Geometry check sheet. Reference: the model listing, model coordinates, mm. Coordinates: 2 decimals unless noted, no trailing zeros. Write each loop counter-clockwise with the first axis right and the second up, starting at its lowest first coordinate (ties: lowest second). Pieces come first, ordered by that corner, then holes.
from build123d import *

# Parameters (mm, degrees)
BOSS_EXTRUDE1_DEPTH     = 15
CUT_EXTRUDE1_DEPTH      = 30.681644159
CUT_EXTRUDE1_DEPTH_BACK = 30.681644159
SKETCH3_R               = 2.05


with BuildPart() as part:
    # Sketch2 → Boss-Extrude1 (new body)
    with BuildSketch(Plane(origin=(0, 0, 0), x_dir=(1, 0, 0), z_dir=(0, 1, 0))):
        with BuildLine():
            Line((-16, 20), (16, 20))
            Line((16, 20), (16, 0))
            Line((16, 0), (9.075, 0))
            ThreePointArc((9.075, 0), (0, 9.075), (-9.075, 0))
            Line((-9.075, 0), (-16, 0))
            Line((-16, 0), (-16, 20))
        make_face()
    extrude(amount=BOSS_EXTRUDE1_DEPTH)

    # Sketch3 → Cut-Extrude1 (cut, two sides: drawn at the far end of the back side and taken through both)
    with BuildSketch(Plane(origin=(0, 0, -20), x_dir=(-1, 0, 0), z_dir=(0, 0, -1)).offset(-CUT_EXTRUDE1_DEPTH_BACK)):
        with Locations((-12.75, 7.5)):
            Circle(SKETCH3_R)
        with Locations((12.75, 7.5)):
            Circle(SKETCH3_R)
    extrude(amount=CUT_EXTRUDE1_DEPTH + CUT_EXTRUDE1_DEPTH_BACK, mode=Mode.SUBTRACT)


solid = part.part
1. Draft check along X on faces 1 (the flat face through (-16, 7, -10)), 2 (the flat face through (0, 0, -12)), 3 (the cylindrical face through (0.2, 7.395, -9.073)). Enter one of: released by +X, released by -X, zero draft, split by the parting line, or undercut.
Computed values:
face 1: released by -X
face 2: zero draft
face 3: undercut
2. Sectioned sample at B-B, the plane x = 12.75. Record the boundary of the cut face in (y, z).
Computed values:
outline: (0, -20) - (5.45, -20) - (5.45, 0) - (0, 0) - close; (9.55, -20) - (15, -20) - (15, 0) - (9.55, 0) - close
3. Sectioned sample at A-A, the plane z = -7. Record the boundary of the cut face in (x, y).
Computed values:
outline: (-16, 0) - (-5.78, 0) - (-5.78, 15) - (-16, 15) - close; (5.78, 0) - (16, 0) - (16, 15) - (5.78, 15) - close; hole circle Ø4.1 at (-12.75, 7.5); hole circle Ø4.1 at (12.75, 7.5)
4. Gauge pin test, flat end, axial feed: pin 1 Ø6 at (x, z) = (1.5, -3.5) entering from +Y. Record the tip position at first contact, or that the pin passes through.
Computed values:
pin 1: passes through
5. Sectioned sample at C-C, the plane y = 7.5. Record the boundary of the cut face in (x, z) (3 decimals).
Computed values:
outline: (-16, -20) - (-14.8, -20) - (-14.8, 0) - (-16, 0) - close; (-10.7, -20) - (10.7, -20) - (10.7, 0) - (9.075, 0) arc R9.075 cw to (-9.075, 0) - (-10.7, 0) - close; (14.8, -20) - (16, -20) - (16, 0) - (14.8, 0) - close
6. Sectioned sample at D-D, the plane z = -14.5. Record the boundary of the cut face in (x, y), and give its area (3 significant figures).
Computed values:
outline: (-16, 0) - (16, 0) - (16, 15) - (-16, 15) - close; hole circle Ø4.1 at (-12.75, 7.5); hole circle Ø4.1 at (12.75, 7.5)
area: 454 mm2
7. Thickness scan on line 1 along X through (y, z) = (7.5, -14.5); line 2 along Y through (x, z) = (-12.75, -9); line 3 along X through (y, z) = (6.5, -16). Record the ranges inside material, lowest first.
Computed values:
line 1: x = -16 to -14.8, -10.7 to 10.7, 14.8 to 16
line 2: y = 0 to 5.45, 9.55 to 15
line 3: x = -16 to -14.54, -10.96 to 10.96, 14.54 to 16
